Part model, mm, in its own coordinate system. A direction names the side the tool comes from. Round coordinates to 2 decimals unless told otherwise and drop trailing zeros. Write each loop counter-clockwise with the first axis right and the second up, starting at its lowest first coordinate (ties: lowest second). Pieces come first, ordered by that corner, then holes. Notation, with made-up numbers: (27, 35) -> (86, 35) arc R21 cw to (86, 42) -> close; hole circle Ø3 at (-16, -34). An arc over 180 degrees is marked (long way). Use CSV: the item, a comma, the result in double quotes. Start each with the question number.
(1) Saw through at D-D (x = 86.5). Give the cut face in (y, z).
(2) Two-plate mould, pull along Z, no slides. Class faces 1 (the flat face through (149, 10, 14)), 2 (the flat face through (1.2, 2.54, 11.87)), 3 (the flat face through (-11.616, 2.535, -1.629)): released by +Z, released by -Z, zero draft, split by the parting line, or undercut.
(3) Probe line 1 (Y direction, x = 66, z = -108); line 2 (Z direction, x = 129, y = 3.75); line 3 (X direction, y = 4.25, z = -102.5). List the from-to ranges inside material, lowest first. Write a range as [from, to].
(4) Saw through at A-A (z = -135). Give the cut face in (x, y), plus the area to 3 significant figures.
(5) Drop flat-ended pins along their axis: pin 1 (5 mm diameter, centred on x = 5, z = -135, fed in from -Y); pin 2 (5 mm diameter, centred on x = 5.5, z = -137, fed in from +Y); pin 3 (2.5 mm diameter, centred on x = 68, y = 2.5, fed in from -Z); pin 4 (5 mm diameter, centred on y = 2, z = 0, fed in from -X). Give the stop position or say it passes through.
(6) Saw through at C-C (z = -32). Give the cut face in (x, y), plus the area to 3 significant figures.
(7) Which spindle directions (+Z, -Z, +X, -X, +Y, -Y) get a long thin tool onto all of the face, cutting with end or side? Do faces 4 (the cylindrical face through (9.436, 5.986, -2.693)), 5 (the flat face through (0, 2, -69)), 6 (the cylindrical face through (112.48, 2.46, -140.72)), 7 (the cylindrical face through (134.68, 2.46, -118.33)). Say none if no direction does.
(8) Saw through at B-B (x = 129). Give the cut face in (y, z).
```python
from build123d import *

# Parameters (mm, degrees)
SKETCH1_W                                  = 134
SKETCH1_H                                  = 140
BOSS_EXTRUDE1_DEPTH                        = 5
BOSS_EXTRUDE3_DEPTH                        = 5
SKETCH3_R                                  = 5
BOSS_EXTRUDE4_DEPTH                        = 5
HOLE1_OUTLINE_R                            = 2.5
HOLE1_DEPTH                                = 10
SKETCH6_R                                  = 5
BOSS_EXTRUDE5_DEPTH                        = 2
HOLE2_OUTLINE_R                            = 2.15
HOLE2_DEPTH                                = 7
MIRROR1_AT_THE_SECOND_PLANE_COPY_1_DEPTH   = 5
MIRROR1_AT_THE_SECOND_PLANE_COPY_2_SKETC_R = 5
MIRROR1_AT_THE_SECOND_PLANE_COPY_2_DEPTH   = 5
MIRROR1_AT_THE_SECOND_PLANE_COPY_3_SKETC_R = 2.5
MIRROR1_AT_THE_SECOND_PLANE_COPY_3_DEPTH   = 10
MIRROR1_AT_THE_SECOND_PLANE_COPY_4_SKETC_R = 5
MIRROR1_AT_THE_SECOND_PLANE_COPY_4_DEPTH   = 2
MIRROR1_AT_THE_SECOND_PLANE_COPY_5_SKETC_R = 2.15
MIRROR1_AT_THE_SECOND_PLANE_COPY_5_DEPTH   = 7
CUT_EXTRUDE_THIN1_DEPTH                    = 232.199441913
MIRROR2_AT_THE_SECOND_PLANE_COPY_1_DEPTH   = 232.199441913
FILLET1_R                                  = 20


# Read off the part's stored shape, not the designer's step: Hole1, Hole2
with BuildPart() as part:
    # Sketch1 → Boss-Extrude1 (new body)
    with BuildSketch(Plane(origin=(0, 0, 0), x_dir=(1, 0, 0), z_dir=(0, 1, 0))):
        with Locations((67, 70)):
            Rectangle(SKETCH1_W, SKETCH1_H)
    extrude(amount=BOSS_EXTRUDE1_DEPTH)

    # Sketch2 → Boss-Extrude3 (add)
    with BuildSketch(Plane(origin=(0, 5, 0), x_dir=(1, 0, 0), z_dir=(0, 1, 0))):
        with BuildLine():
            Line((0, 118.595175856), (-24.35045716, 150.329309467))
            ThreePointArc((-24.35045716, 150.329309467), (-23.487991569, 163.487991569), (-10.329309467, 164.35045716))
            Line((-10.329309467, 164.35045716), (21.404824144, 140))
            Line((21.404824144, 140), (0, 140))
            Line((0, 140), (0, 118.595175856))
        make_face()
    boss_extrude3 = extrude(amount=-BOSS_EXTRUDE3_DEPTH)

    # Sketch3 → Boss-Extrude4 (add)
    with BuildSketch(Plane(origin=(0, 5, 0), x_dir=(1, 0, 0), z_dir=(0, 1, 0))):
        with Locations(Location((-16.416923757, 156.416923757, 0), (0, 0, 90))):
            Circle(SKETCH3_R)
    boss_extrude4 = extrude(amount=BOSS_EXTRUDE4_DEPTH)

    # Hole1 outline → Hole1 (cut)
    with BuildSketch(Plane(origin=(0, 0, 0), x_dir=(1, 0, 0), z_dir=(0, 1, 0))):
        with Locations((-16.416923757, 156.416923757)):
            Circle(HOLE1_OUTLINE_R)
    hole1 = extrude(amount=HOLE1_DEPTH, mode=Mode.SUBTRACT)

    # Sketch6 → Boss-Extrude5 (add)
    with BuildSketch(Plane(origin=(0, 5, 0), x_dir=(1, 0, 0), z_dir=(0, 1, 0))):
        with Locations(Location((5, 135, 0), (0, 0, 90))):
            Circle(SKETCH6_R)
    boss_extrude5 = extrude(amount=BOSS_EXTRUDE5_DEPTH)

    # Hole2 outline → Hole2 (cut)
    with BuildSketch(Plane(origin=(0, 0, 0), x_dir=(1, 0, 0), z_dir=(0, 1, 0))):
        with Locations((5, 135)):
            Circle(HOLE2_OUTLINE_R)
    hole2 = extrude(amount=HOLE2_DEPTH, mode=Mode.SUBTRACT)

    # Mirror1: Boss-Extrude3, Boss-Extrude4, Hole1, Boss-Extrude5, Hole2 across plane
    add(boss_extrude3.mirror(Plane.XY.offset(-70)))
    add(boss_extrude4.mirror(Plane.XY.offset(-70)))
    add(hole1.mirror(Plane.XY.offset(-70)), mode=Mode.SUBTRACT)
    add(boss_extrude5.mirror(Plane.XY.offset(-70)))
    add(hole2.mirror(Plane.XY.offset(-70)), mode=Mode.SUBTRACT)

    # Mirror1 at the second plane: Boss-Extrude3, Boss-Extrude4, Hole1, Boss-Extrude5, Hole2 across plane
    add(boss_extrude3.mirror(Plane.ZY.offset(-67)))
    add(boss_extrude4.mirror(Plane.ZY.offset(-67)))
    add(hole1.mirror(Plane.ZY.offset(-67)), mode=Mode.SUBTRACT)
    add(boss_extrude5.mirror(Plane.ZY.offset(-67)))
    add(hole2.mirror(Plane.ZY.offset(-67)), mode=Mode.SUBTRACT)

    # Mirror1 at the second plane copy 1 sketc → Mirror1 at the second plane copy 1 (add)
    with BuildSketch(Plane(origin=(134, 5, -140), x_dir=(-1, 0, 0), z_dir=(0, 1, 0))):
        with BuildLine():
            Line((0, 118.595175856), (-24.35045716, 150.329309467))
            ThreePointArc((-24.35045716, 150.329309467), (-23.487991569, 163.487991569), (-10.329309467, 164.35045716))
            Line((-10.329309467, 164.35045716), (21.404824144, 140))
            Line((21.404824144, 140), (0, 140))
            Line((0, 140), (0, 118.595175856))
        make_face()
    extrude(amount=-MIRROR1_AT_THE_SECOND_PLANE_COPY_1_DEPTH)

    # Mirror1 at the second plane copy 2 sketc → Mirror1 at the second plane copy 2 (add)
    with BuildSketch(Plane(origin=(134, 5, -140), x_dir=(-1, 0, 0), z_dir=(0, 1, 0))):
        with Locations(Location((-16.416923757, 156.416923757, 0), (0, 0, 90))):
            Circle(MIRROR1_AT_THE_SECOND_PLANE_COPY_2_SKETC_R)
    extrude(amount=MIRROR1_AT_THE_SECOND_PLANE_COPY_2_DEPTH)

    # Mirror1 at the second plane copy 3 sketc → Mirror1 at the second plane copy 3 (cut)
    with BuildSketch(Plane(origin=(134, 0, -140), x_dir=(-1, 0, 0), z_dir=(0, 1, 0))):
        with Locations((-16.416923757, 156.416923757)):
            Circle(MIRROR1_AT_THE_SECOND_PLANE_COPY_3_SKETC_R)
    extrude(amount=MIRROR1_AT_THE_SECOND_PLANE_COPY_3_DEPTH, mode=Mode.SUBTRACT)

    # Mirror1 at the second plane copy 4 sketc → Mirror1 at the second plane copy 4 (add)
    with BuildSketch(Plane(origin=(134, 5, -140), x_dir=(-1, 0, 0), z_dir=(0, 1, 0))):
        with Locations(Location((5, 135, 0), (0, 0, 90))):
            Circle(MIRROR1_AT_THE_SECOND_PLANE_COPY_4_SKETC_R)
    extrude(amount=MIRROR1_AT_THE_SECOND_PLANE_COPY_4_DEPTH)

    # Mirror1 at the second plane copy 5 sketc → Mirror1 at the second plane copy 5 (cut)
    with BuildSketch(Plane(origin=(134, 0, -140), x_dir=(-1, 0, 0), z_dir=(0, 1, 0))):
        with Locations((5, 135)):
            Circle(MIRROR1_AT_THE_SECOND_PLANE_COPY_5_SKETC_R)
    extrude(amount=MIRROR1_AT_THE_SECOND_PLANE_COPY_5_DEPTH, mode=Mode.SUBTRACT)

    # Sketch9 → Cut-Extrude-Thin1 (cut, symmetric)
    with BuildSketch(Plane(origin=(0, 5, 0), x_dir=(1, 0, 0), z_dir=(0, 1, 0))):
        with BuildLine():
            Line((0, 118.595175856), (-20.728209423, 153.88456993))
            ThreePointArc((-20.728209423, 153.88456993), (-19.952457663, 159.952457663), (-13.88456993, 160.728209423))
            Line((-13.88456993, 160.728209423), (21.404824144, 140))
            Line((21.404824144, 140), (26.4695318, 148.622571331))
            Line((26.4695318, 148.622571331), (-8.819862274, 169.350780755))
            ThreePointArc((-8.819862274, 169.350780755), (-27.023525475, 167.023525475), (-29.350780755, 148.819862274))
            Line((-29.350780755, 148.819862274), (-8.622571331, 113.5304682))
            Line((-8.622571331, 113.5304682), (0, 118.595175856))
        make_face()
    cut_extrude_thin1 = extrude(amount=CUT_EXTRUDE_THIN1_DEPTH, both=True, mode=Mode.SUBTRACT)

    # Mirror2: Cut-Extrude-Thin1 across plane
    add(cut_extrude_thin1.mirror(Plane.ZY.offset(-67)), mode=Mode.SUBTRACT)

    # Mirror2 at the second plane: Cut-Extrude-Thin1 across plane
    add(cut_extrude_thin1.mirror(Plane.XY.offset(-70)), mode=Mode.SUBTRACT)

    # Mirror2 at the second plane copy 1 sketc → Mirror2 at the second plane copy 1 (cut, symmetric)
    with BuildSketch(Plane(origin=(134, 5, -140), x_dir=(-1, 0, 0), z_dir=(0, 1, 0))):
        with BuildLine():
            Line((0, 118.595175856), (-20.728209423, 153.88456993))
            ThreePointArc((-20.728209423, 153.88456993), (-19.952457663, 159.952457663), (-13.88456993, 160.728209423))
            Line((-13.88456993, 160.728209423), (21.404824144, 140))
            Line((21.404824144, 140), (26.4695318, 148.622571331))
            Line((26.4695318, 148.622571331), (-8.819862274, 169.350780755))
            ThreePointArc((-8.819862274, 169.350780755), (-27.023525475, 167.023525475), (-29.350780755, 148.819862274))
            Line((-29.350780755, 148.819862274), (-8.622571331, 113.5304682))
            Line((-8.622571331, 113.5304682), (0, 118.595175856))
        make_face()
    extrude(amount=MIRROR2_AT_THE_SECOND_PLANE_COPY_1_DEPTH, both=True, mode=Mode.SUBTRACT)

    # Fillet1
    fillet1_edges = [part.edges().sort_by_distance(p)[0] for p in [
        (0, 2.5, -118.595175856),
        (21.404824144, 2.5, -140),
        (112.595175856, 2.5, -140),
        (134, 2.5, -118.595175856),
        (21.404824144, 2.5, 0),
        (0, 2.5, -21.404824144),
        (134, 2.5, -21.404824144),
        (112.595175856, 2.5, 0),
    ]]
    fillet(fillet1_edges, radius=FILLET1_R)


solid = part.part
```
Answers:
1,outline,"(0, -140) -> (5, -140) -> (5, 0) -> (0, 0) -> close"
2,face 1,"zero draft"
2,face 2,"released by +Z"
2,face 3,"undercut"
3,line 1,"y = [0, 5]"
3,line 2,"z = [-149.64, -137.15], [-132.85, -7.15], [-2.85, 9.64]"
3,line 3,"x = [0, 134]"
4,outline,"(-9.64, 0) -> (2.85, 0) -> (2.85, 7) -> (0, 7) -> (0, 5) -> (-9.64, 5) -> close; (7.15, 0) -> (126.85, 0) -> (126.85, 7) -> (124, 7) -> (124, 5) -> (10, 5) -> (10, 7) -> (7.15, 7) -> close; (131.15, 0) -> (143.64, 0) -> (143.64, 5) -> (134, 5) -> (134, 7) -> (131.15, 7) -> close"
4,area,"746 mm²"
5,pin 1,"stops at y = 0"
5,pin 2,"stops at y = 7"
5,pin 3,"stops at z = -140"
5,pin 4,"stops at x = -14.04"
6,outline,"(0, 0) -> (134, 0) -> (134, 5) -> (0, 5) -> close"
6,area,"670 mm²"
7,face 4,"+Y"
7,face 5,"-X, +Y, -Y"
7,face 6,"-Z, +Y, -Y"
7,face 7,"+X, +Y, -Y"
8,outline,"(0, -149.64) -> (5, -149.64) -> (5, -140) -> (7, -140) -> (7, -137.15) -> (0, -137.15) -> close; (0, -132.85) -> (7, -132.85) -> (7, -130) -> (5, -130) -> (5, -10) -> (7, -10) -> (7, -7.15) -> (0, -7.15) -> close; (0, -2.85) -> (7, -2.85) -> (7, 0) -> (5, 0) -> (5, 9.64) -> (0, 9.64) -> close"
